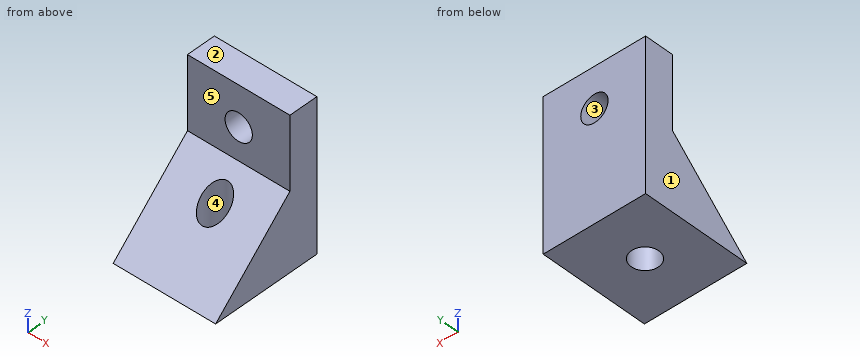
from build123d import *

# Parameters (mm, degrees)
SKETCH1_W               = 15
SKETCH1_H               = 16
BOSS_EXTRUDE1_DEPTH     = 22
CUT_EXTRUDE1_DEPTH      = 22
CUT_EXTRUDE1_DEPTH_BACK = 22
SKETCH6_R               = 2
CUT_EXTRUDE2_DEPTH      = 22
SKETCH7_R               = 2
CUT_EXTRUDE3_DEPTH      = 10


with BuildPart() as part:
    # Sketch1 → Boss-Extrude1 (new body)
    with BuildSketch(Plane.XY):
        Rectangle(SKETCH1_W, SKETCH1_H)
    extrude(amount=BOSS_EXTRUDE1_DEPTH)

    # Sketch4 → Cut-Extrude1 (cut, two sides)
    with BuildSketch(Plane(origin=(0, 0, 0), x_dir=(0, 0, -1), z_dir=(1, 0, 0))) as cut_extrude1_sk:
        Polygon((-22, 3.745733089), (-11.369948947, 3.745733089), (0, -8), (-22, -8), align=None)
    extrude(amount=CUT_EXTRUDE1_DEPTH, mode=Mode.SUBTRACT)
    extrude(cut_extrude1_sk.sketch, amount=-CUT_EXTRUDE1_DEPTH_BACK, mode=Mode.SUBTRACT)

    # Sketch6 → Cut-Extrude2 (cut)
    with BuildSketch(Plane(origin=(0, 8, 0), x_dir=(1, 0, 0), z_dir=(0, 1, 0))):
        with Locations((0, -16.110735895)):
            Circle(SKETCH6_R)
    extrude(amount=-CUT_EXTRUDE2_DEPTH, mode=Mode.SUBTRACT)

    # Sketch7 → Cut-Extrude3 (cut)
    with BuildSketch(Plane(origin=(0, 0, 0), x_dir=(-1, 0, 0), z_dir=(0, 0, -1))):
        Circle(SKETCH7_R)
    extrude(amount=-CUT_EXTRUDE3_DEPTH, mode=Mode.SUBTRACT)


solid = part.part
Model file for the job. Use its own axes, mm. Face numbers are marked on the shaded views. A direction names the side the tool comes from. Round coordinates to 2 decimals unless told otherwise and drop trailing zeros. Order: outer loops, then holes, each group sorted by start corner. A loop starts at its lowest first (then second) coordinate and runs counter-clockwise, first axis right, second up.
(1) Band-saw the part on C-C (z = 14.75). List the corners of the cut face in (x, y), then the cut area to 3 significant figures.
(2) Drill centre lines: line 1 (Z direction, x = 0, y = 5.15); line 2 (X direction, y = 0, z = 4.5); line 3 (Y direction, x = 5, z = 18.5). Where is each one in solid material? Low to high.
(3) Band-saw the part on D-D (z = 2.25). List the corners of the cut face in (x, y).
(4) 3-axis set-ups, long thin cutter, end or side, ignore diameter. For the marked faces 4 and 5: which of +Z, -Z, +X, -X, +Y, -Y reach the whole face in a straight line?
(5) Pull direction X, two halves, no side cores. Call the marked faces 1, 2 and 3: released by +X, released by -X, zero draft, split by the parting line, or undercut.
(6) Pin check, flat tips, straight feed: pin 1 (3.5 mm diameter, centred on x = 0, y = 0, fed in from -Z); pin 2 (5.5 mm diameter, centred on x = -1.5, z = 18.5, fed in from -Y); pin 3 (2 mm diameter, centred on x = -4, y = -4, fed in from +Z). Stop position of each tip, or through.
(7) Band-saw the part on A-A (y = 1). List the corners of the cut face in (x, z).
(8) Band-saw the part on B-B (x = 4.5). List the corners of the cut face in (y, z), then the cut area to 3 significant figures.
Verdict:
1. outline: (-7.5, 3.75) - (-1.47, 3.75) - (-1.47, 8) - (-7.5, 8) - close; (1.47, 3.75) - (7.5, 3.75) - (7.5, 8) - (1.47, 8) - close
1. area: 51.3 mm2
2. line 1: z = 0 to 14.11, 18.11 to 22
2. line 2: x = -7.5 to -2, 2 to 7.5
2. line 3: y = 3.75 to 8
3. outline: (-7.5, -5.68) - (7.5, -5.68) - (7.5, 8) - (-7.5, 8) - close; hole circle Ø4 at (0, 0)
4. face 4: +Z, -Z
4. face 5: +Z, +X, -X, -Y
5. face 1: released by -X
5. face 2: zero draft
5. face 3: undercut
6. pin 1: passes through
6. pin 2: stops at y = 3.75
6. pin 3: stops at z = 4.84
7. outline: (-7.5, 0) - (-1.73, 0) - (-1.73, 8.71) - (-7.5, 8.71) - close; (1.73, 0) - (7.5, 0) - (7.5, 8.71) - (1.73, 8.71) - close
8. outline: (-8, 0) - (8, 0) - (8, 22) - (3.75, 22) - (3.75, 11.37) - close
8. area: 160 mm2
